Read the model definition and answer for the solid it produces. Units are mm, in the model's axes. A direction names the side the tool comes from. Round coordinates to 2 decimals unless told otherwise and drop trailing zeros. Order: outer loops, then holes, each group sorted by start corner. A loop starts at its lowest first (then second) coordinate and runs counter-clockwise, first axis right, second up. Notation, with made-up numbers: (-16, 12) - (30, 12) arc R17 ccw to (30, 17) - close; hole circle Ø9 at (-32, 4.5). An arc over 180 degrees is marked (long way). Answer as a JSON object with one key per item and string values. Group by question number.
Q1. A tool of negligible diameter and unlimited length cuts with its end or side. For faces 1 (the flat face through (38, 7, 1)), 2 (the flat face through (38, 6, 0)), from which of +Z, -Z, +X, -X, +Y, -Y can it reach the whole face along a straight path? Write none if from no direction.
Q2. Given pin 1 Ø10 at (x, z) = (47.5, 53.5) entering from +Y; pin 2 Ø1.5 at (x, y) = (62, 7) entering from +Z, each flat-ended and moving along its own axis, determine where each tip first touches the part or whether it passes through.
Q3. A cutting plane is placed at A-A on x = 45.5. Determine the outline of the cut face in (y, z), and give its area (3 significant figures).
Q4. Consider line 1 (Y direction, x = 15, z = 21). Determine where the line is inside the solid, lowest interval first.
Q5. A cutting plane is placed at B-B on y = 6. Determine the outline of the cut face in (x, z), and give its area (3 significant figures).
```python
from build123d import *

# Parameters (mm, degrees)
F1_DEPTH = 78
F2_R     = 4
F3_R     = 1


# Not quite as in the source:
# - two fillets or chamfers of one size are made in one step


with BuildPart() as f1:
    # F0 (on Right) → F1 (new body)
    with BuildSketch(Plane.YZ):
        Polygon((0, 78), (0, 0), (12, 0), (12, 1), (1, 1), (1, 78), align=None)
    extrude(amount=F1_DEPTH)

    # F2
    f2_edges = [f1.edges().sort_by_distance(p)[0] for p in [
        (78, 0.5, 78),
    ]]
    fillet(f2_edges, radius=F2_R)

    # F3
    f3_edges = [f1.edges().sort_by_distance(p)[0] for p in [
        (0, 12, 0.5),
        (39, 0, 0),
        (78, 12, 0.5),
    ]]
    fillet(f3_edges, radius=F3_R)


solid = f1.part
```
Result set:
{
 "1": {"face 1": "+Z, +X, -X, +Y", "face 2": "-Z, +X, -X, +Y, -Y"},
 "2": {"pin 1": "stops at y = 1", "pin 2": "stops at z = 1"},
 "3": {"outline": "(0, 1) arc R1 ccw to (1, 0) - (12, 0) - (12, 1) - (1, 1) - (1, 78) - (0, 78) - close", "area": "88.8 mm²"},
 "4": {"line 1": "y = 0 to 1"},
 "5": {"outline": "(0, 0) - (78, 0) - (78, 1) - (0, 1) - close", "area": "78.0 mm²"}
}
